```python
from build123d import *

# Parameters (mm, degrees)
SKETCH1_W                = 85.725
SKETCH1_H                = 66.675
BOSS_EXTRUDE1_DEPTH      = 6.858
FILLET1_R                = 2.54
SKETCH2_W                = 69.596
SKETCH2_H                = 50.419
CUT_EXTRUDE1_DEPTH       = 3.81
FILLET2_R                = 0.381
SKETCH3_R                = 0.7239
CUT_EXTRUDE2_DEPTH       = 3.556
M3_CLEARANCE_HOLE1_D     = 3.4
M3_CLEARANCE_HOLE1_DEPTH = 6.858
SKETCH6_W                = 46.393114838
SKETCH6_H                = 46.99
CUT_EXTRUDE3_DEPTH       = 3.81
FILLET3_R                = 0.381
FILLET4_R                = 1.27


with BuildPart() as part:
    # Sketch1 → Boss-Extrude1 (new body)
    with BuildSketch(Plane(origin=(0, 0, 0), x_dir=(1, 0, 0), z_dir=(0, 1, 0))):
        Rectangle(SKETCH1_W, SKETCH1_H)
    extrude(amount=BOSS_EXTRUDE1_DEPTH)

    # Fillet1
    fillet1_edges = [part.edges().sort_by_distance(p)[0] for p in [
        (42.8625, 3.429, 33.3375),
        (-42.8625, 3.429, 33.3375),
        (-42.8625, 3.429, -33.3375),
        (42.8625, 3.429, -33.3375),
    ]]
    fillet(fillet1_edges, radius=FILLET1_R)

    # Sketch2 → Cut-Extrude1 (cut)
    with BuildSketch(Plane(origin=(0, 6.858, 0), x_dir=(1, 0, 0), z_dir=(0, 1, 0))):
        Rectangle(SKETCH2_W, SKETCH2_H)
    extrude(amount=-CUT_EXTRUDE1_DEPTH, mode=Mode.SUBTRACT)

    # Fillet2
    fillet2_edges = [part.edges().sort_by_distance(p)[0] for p in [
        (-34.798, 4.953, 25.2095),
        (-34.798, 4.953, -25.2095),
        (34.798, 4.953, -25.2095),
        (34.798, 4.953, 25.2095),
    ]]
    fillet(fillet2_edges, radius=FILLET2_R)

    # Sketch3 → Cut-Extrude2 (cut)
    with BuildSketch(Plane(origin=(0, 3.048, 0), x_dir=(1, 0, 0), z_dir=(0, 1, 0))):
        with Locations(Location((-33.9725, 24.4729, 0), (0, 0, 270))):
            Circle(SKETCH3_R)
        with Locations(Location((33.9725, 24.4729, 0), (0, 0, 270))):
            Circle(SKETCH3_R)
        with Locations(Location((33.9725, -24.4729, 0), (0, 0, 270))):
            Circle(SKETCH3_R)
        with Locations(Location((-33.9725, -24.4729, 0), (0, 0, 270))):
            Circle(SKETCH3_R)
    extrude(amount=-CUT_EXTRUDE2_DEPTH, mode=Mode.SUBTRACT)

    # M3 Clearance Hole1
    with Locations(Plane(origin=(0, 0, 0), x_dir=(-1, 0, 0), z_dir=(0, -1, 0))):
        with Locations((-39.0525, 28.8925), (0, 0), (39.0525, 28.8925), (-39.0525, -28.8925), (39.0525, -28.8925)):
            Hole(M3_CLEARANCE_HOLE1_D / 2, depth=M3_CLEARANCE_HOLE1_DEPTH)

    # Sketch6 → Cut-Extrude3 (cut)
    with BuildSketch(Plane(origin=(0, 6.858, 0), x_dir=(1, 0, 0), z_dir=(0, 1, 0))):
        with Locations((-42.86502452, 0)):
            Rectangle(SKETCH6_W, SKETCH6_H)
    extrude(amount=-CUT_EXTRUDE3_DEPTH, mode=Mode.SUBTRACT)

    # Fillet3
    fillet3_edges = [part.edges().sort_by_distance(p)[0] for p in [
        (-34.798, 4.953, -23.495),
        (-34.798, 4.953, 23.495),
    ]]
    fillet(fillet3_edges, radius=FILLET3_R)

    # Fillet4
    fillet4_edges = [part.edges().sort_by_distance(p)[0] for p in [
        (-42.8625, 4.953, -23.495),
        (-42.8625, 4.953, 23.495),
    ]]
    fillet(fillet4_edges, radius=FILLET4_R)


solid = part.part
```
Could you check a few things on this model? Use its own coordinates, in mm. A direction names the side the tool comes from. Round coordinates to 2 decimals unless told otherwise and drop trailing zeros. Write each loop counter-clockwise with the first axis right and the second up, starting at its lowest first coordinate (ties: lowest second). Pieces come first, ordered by that corner, then holes. Notation, with made-up numbers: M 56,-2 L 79,-2 A21 cw 79,2 Z; hole C -25.5,58 d3. An arc over 180 degrees is marked long. Answer in a Markdown table with one row per item. Add a question column.
Q1. Will these pins go through, and if not, where does the flat tip stop? pin 1 Ø3 at (y, z) = (5, 7) entering from -X; pin 2 Ø12 at (x, z) = (-2, 20) entering from +Y; pin 3 Ø2.5 at (x, z) = (0, 0) entering from -Y.
Q2. Imagine slicing it at B-B (x = 0). Please give me the cut outline in (y, z), then the cut area to 3 significant figures.
Q3. Imagine slicing it at A-A (z = 0). Please give me the cut outline in (x, y), then the cut area to 3 significant figures.
Q4. If we mould it in two halves opening along Z, with no side actions, what happens to faces 4 (the flat face through (-42.862, 2, 0)), 5 (the cylindrical face through (-40.305, 3.477, 27.744)), 6 (the flat face through (-1, 3, -33.338))? For each: +Z half, -Z half, draft (parallel to the pull), parting line (faces both ways), or undercut.
Q5. Imagine slicing it at D-D (x = -27.5). Please give me the cut outline in (y, z).
Q6. Imagine slicing it at C-C (y = 4.5). Please give me the cut outline in (x, z) (1 decimal).
Q7. On a 3-axis mill with a long thin cutter (end or side, diameter ignored), from which of +Z, -Z, +X, -X, +Y, -Y can I reach the whole of each face in a straight line? I mean faces 1 (the flat face through (-38, 5, 23.495)), 2 (the flat face through (0, 5, 25.21)), 3 (the flat face through (42.862, 3, 0)). Say none if no direction works.
Q8. If I drill on line 1 (X direction, y = 0.5, z = -29); line 2 (Z direction, x = 18.5, y = 4.5); line 3 (Y direction, x = -0.5, z = -9.5), over which ranges is the centre line in solid material (lowest first)? Write a range as from..to.
Values:
| question | item | result |
|---|---|---|
| 1 | pin 1 | x = 34.8 |
| 1 | pin 2 | y = 6.86 |
| 1 | pin 3 | through |
| 2 | outline | M 0,-33.34 L 6.86,-33.34 L 6.86,-25.21 L 3.05,-25.21 L 3.05,-1.7 L 0,-1.7 Z; M 0,1.7 L 3.05,1.7 L 3.05,25.21 L 6.86,25.21 L 6.86,33.34 L 0,33.34 Z |
| 2 | area | 255 mm^2 |
| 3 | outline | M -42.86,0 L -1.7,0 L -1.7,3.05 L -42.86,3.05 Z; M 1.7,0 L 42.86,0 L 42.86,6.86 L 34.8,6.86 L 34.8,3.05 L 1.7,3.05 Z |
| 3 | area | 282 mm^2 |
| 4 | face 4 | draft |
| 4 | face 5 | undercut |
| 4 | face 6 | -Z half |
| 5 | outline | M 0,-33.34 L 6.86,-33.34 L 6.86,-25.21 L 3.05,-25.21 L 3.05,25.21 L 6.86,25.21 L 6.86,33.34 L 0,33.34 Z |
| 6 | outline | M -42.9,-30.8 A2.5 ccw -40.3,-33.3 L 40.3,-33.3 A2.5 ccw 42.9,-30.8 L 42.9,30.8 A2.5 ccw 40.3,33.3 L -40.3,33.3 A2.5 ccw -42.9,30.8 L -42.9,24.8 A1.3 ccw -41.6,23.5 L -35.2,23.5 A0.4 ccw -34.8,23.9 L -34.8,24.8 A0.4 cw -34.4,25.2 L 34.4,25.2 A0.4 cw 34.8,24.8 L 34.8,-24.8 A0.4 cw 34.4,-25.2 L -34.4,-25.2 A0.4 cw -34.8,-24.8 L -34.8,-23.9 A0.4 ccw -35.2,-23.5 L -41.6,-23.5 A1.3 ccw -42.9,-24.8 Z; hole C -39.1,-28.9 d3.4; hole C -39.1,28.9 d3.4; hole C 39.1,-28.9 d3.4; hole C 39.1,28.9 d3.4 |
| 7 | face 1 | -X, +Y |
| 7 | face 2 | +Y |
| 7 | face 3 | +Z, -Z, +X, +Y, -Y |
| 8 | line 1 | -42.86..-40.75, -37.36..37.36, 40.75..42.86 |
| 8 | line 2 | -33.34..-25.21, 25.21..33.34 |
| 8 | line 3 | 0..3.05 |
